Answer from the drawing. Dimensions are ordinates in mm from the lowest x, y and z of the part. A direction names the side the tool comes from. Give positions to 0.01 mm unless a question says otherwise; leave off trailing zeros. Order: outer loops, then holes, each group sorted by start corner. A loop starts at its lowest first (then second) coordinate and runs counter-clockwise, first axis right, second up. Notation, with made-up numbers: (73.25, 80.5) - (131.25, 80.5) arc R14 cw to (131.25, 94.5) - close; hole circle Ø1 at (25.5, -5.75). An arc over 180 degrees is marked (long way). Use a Markdown table: item, result. Add a question column.
1) Find section B-B, the plane x = 4.6. Determine the outline of the cut face in (y, z), plus the area to 3 significant figures.
2) Flat-ended cylindrical pins translate along their axes: pin 1 (3 mm diameter, centred on x = 7, z = 7, fed in from +Y); pin 2 (3 mm diameter, centred on x = 8, y = 6, fed in from -Z); pin 3 (0.6 mm diameter, centred on x = 4.5, y = 2, fed in from -Z); pin 4 (1.5 mm diameter, centred on x = 8, y = 8, fed in from -Z). Find the tip coordinate at first contact, or state that the pin passes through.
3) Straight lines are drawn through the part: line 1 (Y direction, x = 2.5, z = 2.5); line 2 (Z direction, x = 4.75, y = 6); line 3 (Y direction, x = 1.25, z = 3.25). For each, find the intervals that lie inside material, in ascending order.
4) Find section D-D, the plane z = 2. Determine the outline of the cut face in (x, y).
5) For the marked faces 4, 5, 6 and 7, determine the directions among +Z, -Z, +X, -X, +Y, -Y from which every point of the face is accessible in a straight line to the end or side of a thin tool.
6) The mould has two halves that part along Z. Classify the marked faces 1, 2 and 3: released by +Z, released by -Z, zero draft, split by the parting line, or undercut.
7) Find section A-A, the plane y = 4. Determine the outline of the cut face in (x, z), plus the area to 3 significant figures.
8) Find section C-C, the plane z = 4.6. Determine the outline of the cut face in (x, y).
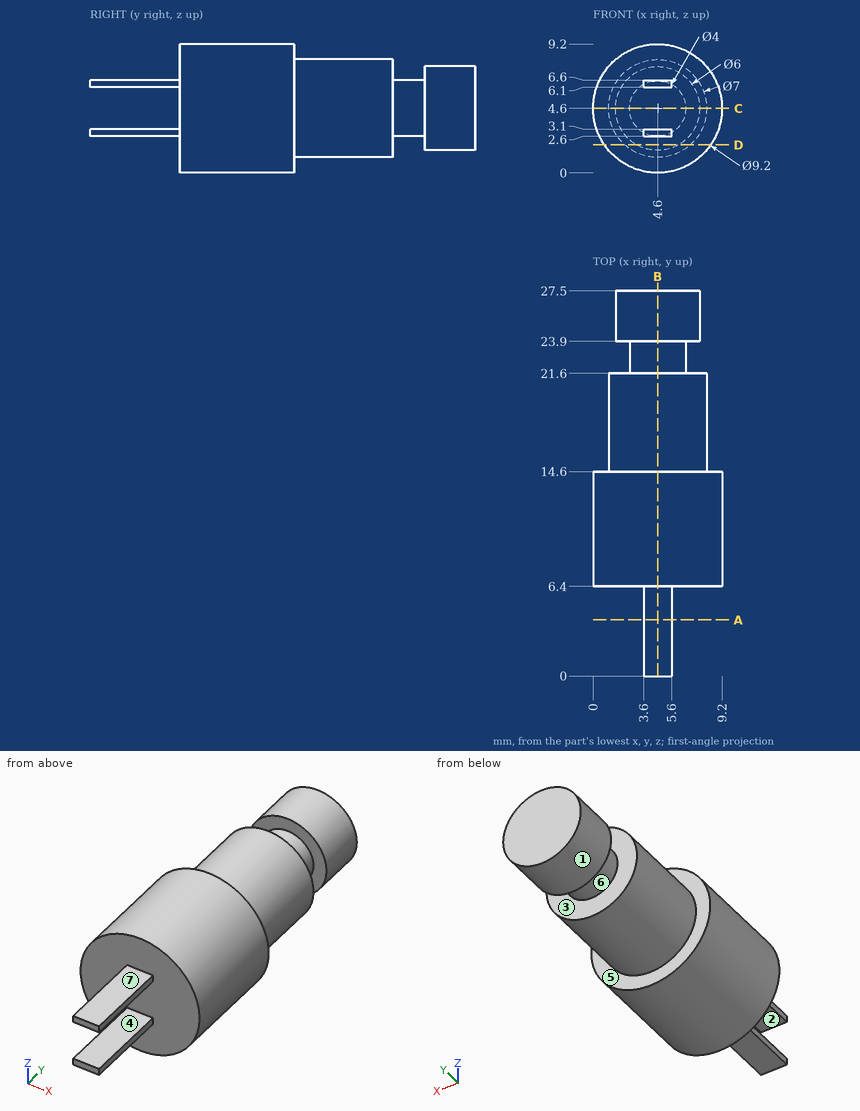
The answers:
| question | item | result |
|---|---|---|
| 1 | outline | (0, 2.6) - (6.4, 2.6) - (6.4, 0) - (14.6, 0) - (14.6, 1.1) - (21.6, 1.1) - (21.6, 2.6) - (23.9, 2.6) - (23.9, 1.6) - (27.5, 1.6) - (27.5, 7.6) - (23.9, 7.6) - (23.9, 6.6) - (21.6, 6.6) - (21.6, 8.1) - (14.6, 8.1) - (14.6, 9.2) - (6.4, 9.2) - (6.4, 6.6) - (0, 6.6) - (0, 6.1) - (6.4, 6.1) - (6.4, 3.1) - (0, 3.1) - close |
| 1 | area | 162 mm2 |
| 2 | pin 1 | y = 27.5 |
| 2 | pin 2 | z = 0.44 |
| 2 | pin 3 | z = 2.6 |
| 2 | pin 4 | z = 0.84 |
| 3 | line 1 | 6.4 to 21.6, 23.9 to 27.5 |
| 3 | line 2 | 2.6 to 3.1, 6.1 to 6.6 |
| 3 | line 3 | 6.4 to 14.6 |
| 4 | outline | (0.81, 6.4) - (8.39, 6.4) - (8.39, 14.6) - (6.94, 14.6) - (6.94, 21.6) - (2.26, 21.6) - (2.26, 14.6) - (0.81, 14.6) - close; (3.1, 23.9) - (6.1, 23.9) - (6.1, 27.5) - (3.1, 27.5) - close |
| 5 | face 4 | +X, -X, -Y |
| 5 | face 5 | +Y |
| 5 | face 6 | none |
| 5 | face 7 | +Z, +X, -X, -Y |
| 6 | face 1 | split by the parting line |
| 6 | face 2 | undercut |
| 6 | face 3 | zero draft |
| 7 | outline | (3.6, 2.6) - (5.6, 2.6) - (5.6, 3.1) - (3.6, 3.1) - close; (3.6, 6.1) - (5.6, 6.1) - (5.6, 6.6) - (3.6, 6.6) - close |
| 7 | area | 2.00 mm2 |
| 8 | outline | (0, 6.4) - (9.2, 6.4) - (9.2, 14.6) - (8.1, 14.6) - (8.1, 21.6) - (6.6, 21.6) - (6.6, 23.9) - (7.6, 23.9) - (7.6, 27.5) - (1.6, 27.5) - (1.6, 23.9) - (2.6, 23.9) - (2.6, 21.6) - (1.1, 21.6) - (1.1, 14.6) - (0, 14.6) - close |
